from build123d import *

# Parameters (mm, degrees)
SKETCH_1_R          = 3
EXTRUDE_1_DEPTH     = 8
SKETCH_3_W          = 12
SKETCH_3_H          = 20
EXTRUDE_2_DEPTH     = 36
SKETCH_8_R          = 10
EXTRUDE_4_DEPTH     = 60
EXTRUDE_4_2_DEPTH   = 60
CUT_EXTRUDE_1_DEPTH = 89
SKETCH_12_W         = 8
SKETCH_12_H         = 20
EXTRUDE_5_DEPTH     = 70
SKETCH_13_W         = 16
SKETCH_13_H         = 35.268464788
CUT_EXTRUDE_2_DEPTH = 140
SKETCH_14_W         = 20
SKETCH_14_H         = 20
EXTRUDE_6_DEPTH     = 40
CUT_EXTRUDE_3_DEPTH = 40
SKETCH_16_W         = 28.583727007
SKETCH_16_H         = 28.583727007
CUT_EXTRUDE_4_DEPTH = 5


with BuildPart() as part:
    # Sketch 1 → Extrude 1 (new body)
    with BuildSketch(Plane(origin=(0, 0, 0), x_dir=(0, 0, -1), z_dir=(1, 0, 0))):
        with BuildLine():
            Line((-18, 0), (-18, 140))
            Line((-18, 140), (18, 140))
            Line((18, 140), (18, 0))
            ThreePointArc((18, 0), (0, -18), (-18, 0))
        make_face()
        Circle(SKETCH_1_R, mode=Mode.SUBTRACT)
    extrude(amount=EXTRUDE_1_DEPTH)

    # Sketch 3 → Extrude 2 (add)
    with BuildSketch(Plane(origin=(0, 0, -18), x_dir=(-1, 0, 0), z_dir=(0, 0, -1))):
        with Locations((-14, 130)):
            Rectangle(SKETCH_3_W, SKETCH_3_H)
    extrude(amount=-EXTRUDE_2_DEPTH)

    # Sketch 10 → Cut-Extrude 1 (cut, through all)
    with BuildSketch(Plane.XY.offset(18)):
        with BuildLine():
            Line((0, 130), (-3.859245882, 130))
            Line((-3.859245882, 130), (-3.859245882, 144.839572577))
            Line((-3.859245882, 144.839572577), (22.991832782, 144.839572577))
            Line((22.991832782, 144.839572577), (22.991832782, 116.883342809))
            Line((22.991832782, 116.883342809), (10, 116.883342809))
            Line((10, 116.883342809), (10, 120))
            ThreePointArc((10, 120), (17.071067812, 137.071067812), (0, 130))
        make_face()
    extrude(amount=-CUT_EXTRUDE_1_DEPTH, mode=Mode.SUBTRACT)



with BuildPart() as body_2:
    # Sketch 8 → Extrude 4 (new body)
    with BuildSketch(Plane(origin=(8, 0, 0), x_dir=(0, 0, -1), z_dir=(1, 0, 0))):
        with Locations((-60, 90)):
            Circle(SKETCH_8_R)
    extrude(amount=EXTRUDE_4_DEPTH)


with BuildPart() as body_3:
    # Sketch 8 → Extrude 4 2 (new body)
    with BuildSketch(Plane(origin=(8, 0, 0), x_dir=(0, 0, -1), z_dir=(1, 0, 0))):
        with Locations((60, 90)):
            Circle(SKETCH_8_R)
    extrude(amount=EXTRUDE_4_2_DEPTH)


with BuildPart() as part_1:
    add(part.part)

    add(body_2.part)  # Extrude 5 merges body 2

    add(body_3.part)  # Extrude 5 merges body 3
    # Sketch 12 → Extrude 5 (add, symmetric)
    with BuildSketch(Plane.XY):
        with Locations((4, 90)):
            Rectangle(SKETCH_12_W, SKETCH_12_H)
    extrude(amount=EXTRUDE_5_DEPTH, both=True)

    # Sketch 13 → Cut-Extrude 2 (cut)
    with BuildSketch(Plane.ZY):
        with Locations((0, 131.634232394)):
            Rectangle(SKETCH_13_W, SKETCH_13_H)
    extrude(amount=-CUT_EXTRUDE_2_DEPTH, mode=Mode.SUBTRACT)

    # Sketch 14 → Extrude 6 (add)
    with BuildSketch(Plane(origin=(8, 0, 0), x_dir=(0, 0, -1), z_dir=(1, 0, 0))):
        with Locations((0, 62)):
            Rectangle(SKETCH_14_W, SKETCH_14_H)
    extrude(amount=EXTRUDE_6_DEPTH)

    # Sketch 15 → Cut-Extrude 3 (cut)
    with BuildSketch(Plane(origin=(0, 0, -10), x_dir=(-1, 0, 0), z_dir=(0, 0, -1))):
        with BuildLine():
            Line((-38, 72), (-54.351268728, 72))
            Line((-54.351268728, 72), (-54.351268728, 52))
            Line((-54.351268728, 52), (-38, 52))
            ThreePointArc((-38, 52), (-48, 62), (-38, 72))
        make_face()
    extrude(amount=-CUT_EXTRUDE_3_DEPTH, mode=Mode.SUBTRACT)

    # Sketch 16 → Cut-Extrude 4 (cut, symmetric)
    with BuildSketch(Plane.XY):
        with Locations((37.291863503, 60.532166911)):
            Rectangle(SKETCH_16_W, SKETCH_16_H)
    extrude(amount=CUT_EXTRUDE_4_DEPTH, both=True, mode=Mode.SUBTRACT)


solid = part_1.part
CAD build for the part. Positions are in the model's coordinates, mm. A direction names the side the tool comes from. Round coordinates to 2 decimals unless told otherwise and drop trailing zeros. Order: outer loops, then holes, each group sorted by start corner. A loop starts at its lowest first (then second) coordinate and runs counter-clockwise, first axis right, second up. Notation, with made-up numbers: (64, 42.25) -> (106, 42.25) arc R22 ccw to (106, 69.25) -> close; hole circle Ø10 at (17.5, 1.25). An arc over 180 degrees is marked (long way). Write item = value, one per line. Start each with the question number.
(1) Cut at A-A, the plane x = 28.5. List the corners of the cut face in (y, z).
(2) Cut at B-B, the plane x = 51.5. List the corners of the cut face in (y, z), then the cut area to 3 significant figures.
(3) Pin check, flat tips, straight feed: P1, Ø6, axis at x = 28, y = 64.5, coming from the +Z side; P2, Ø4, axis at x = 3, z = 46.5, coming from the -Y side; P3, Ø6, axis at x = 5, y = 125, coming from the +Z side; P4, Ø1.5, axis at x = 42.5, z = 11, coming from the +Y side. Stop position of each tip, or through.
(4) Probe line 1 (Z direction, x = 35, y = 89.5); line 2 (Y direction, x = 4.25, z = 0); line 3 (X direction, y = 28, z = 3.5). List the from-to ranges inside material, lowest first. Write a range as [from, to].
(5) Which spindle directions (+Z, -Z, +X, -X, +Y, -Y) get a long thin tool onto all of the face, cutting with end or side? Do faces 1 (the flat face through (4, 41, -18)), 2 (the flat face through (4, 41, 18)), 3 (the flat face through (19, 52, 0)), 4 (the cylindrical face through (37.58, 96.76, -52.63)). Say none if no direction does.
(6) Cut at C-C, the plane z = 0.5. List the corners of the cut face in (x, y), then the cut area to 3 significant figures.
(7) Cut at D-D, the plane y = 62. List the corners of the cut face in (x, z).
(8) Pull direction Z, two halves, no side cores. Call faces 5 (the cylindrical face through (37.58, 96.76, 67.37)), 6 (the cylindrical face through (48, 62, 7)), 7 (the flat face through (8, 125, 18)): released by +Z, released by -Z, zero draft, split by the parting line, or undercut.
Model answer:
q1.outline = (52, -10) -> (72, -10) -> (72, -5) -> (52, -5) -> close; (52, 5) -> (72, 5) -> (72, 10) -> (52, 10) -> close; circle Ø20 at (90, -60); circle Ø20 at (90, 60)
q2.outline = circle Ø20 at (90, -60); circle Ø20 at (90, 60)
q2.area = 628 mm2
q3.P1 = 10
q3.P2 = 80
q3.P3 = 18
q3.P4 = through
q4.line_1 = [-69.99, -50.01], [50.01, 69.99]
q4.line_2 = [-18, -3], [3, 114]
q4.line_3 = [0, 8]
q5.face_1 = -Z, +X, -X, -Y
q5.face_2 = +Z, +X, -X, -Y
q5.face_3 = +Z, -Z, +X, -Y
q5.face_4 = +X
q6.outline = (0, -17.99) -> (8, -17.99) -> (8, -2.96) -> (0, -2.96) -> close; (0, 2.96) -> (8, 2.96) -> (8, 52) -> (23, 52) -> (23, 72) -> (8, 72) -> (8, 114) -> (0, 114) -> close
q6.area = 1,310 mm2
q7.outline = (0, -18) -> (8, -18) -> (8, -10) -> (48, -10) -> (48, -5) -> (23, -5) -> (23, 5) -> (48, 5) -> (48, 10) -> (8, 10) -> (8, 18) -> (0, 18) -> close
q8.face_5 = undercut
q8.face_6 = zero draft
q8.face_7 = released by +Z
